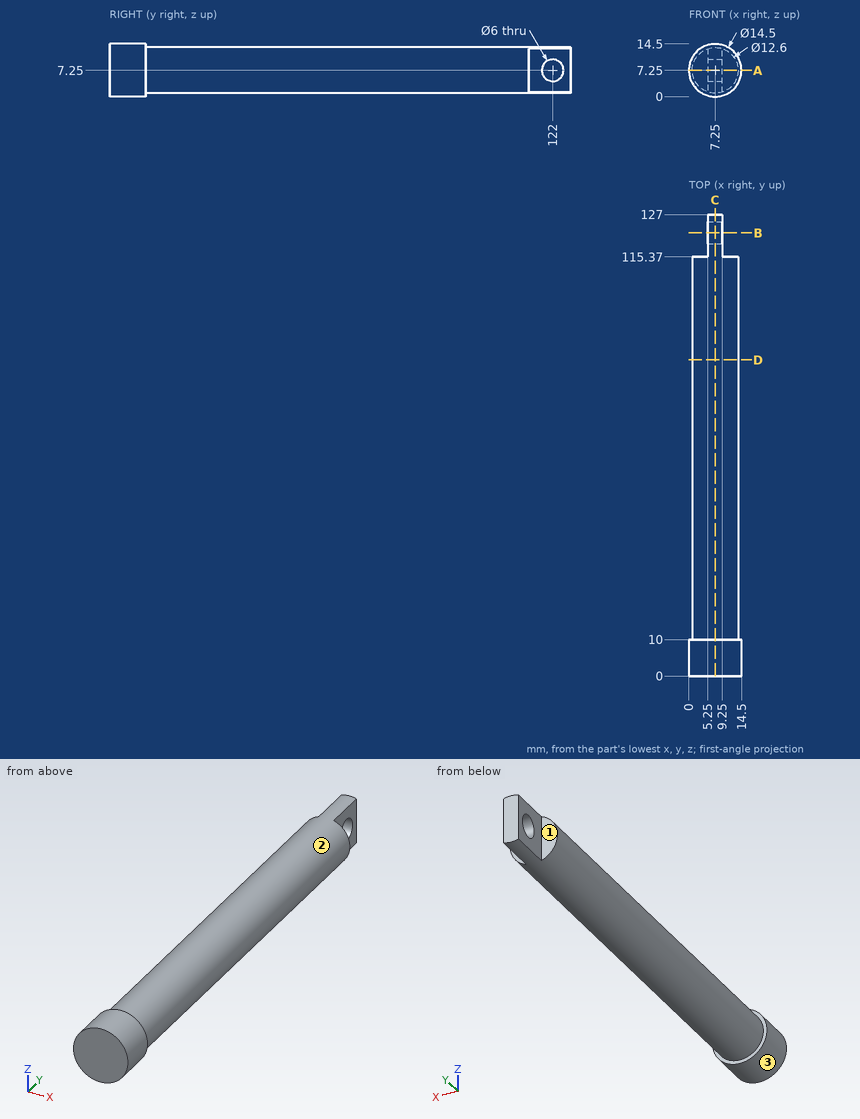
Geometry: see drawing. Coordinates: mm, zero at the bounding-box minimum. A direction names the side the tool comes from. Coordinates: 2 decimals unless noted, no trailing zeros. Loops run counter-clockwise (first coordinate to the right, second up) from the corner with the lowest first, then second, coordinate; pieces in that order, holes last. Notation, with made-up numbers: (46, 19.25) - (69, 19.25) arc R36 cw to (69, 55.25) - close; hole circle Ø2 at (0.25, -20.75). An arc over 180 degrees is marked (long way). Answer as CSV lines item,"result".
1. Section A-A (z = 7.25). Return loops of the section in (x, y).
Established:
outline,"(0, 0) - (14.5, 0) - (14.5, 10) - (13.55, 10) - (13.55, 115.37) - (9.25, 115.37) - (9.25, 119) - (5.25, 119) - (5.25, 115.37) - (0.95, 115.37) - (0.95, 10) - (0, 10) - close; (5.25, 125) - (9.25, 125) - (9.25, 127) - (5.25, 127) - close"
2. Contact query for flat-ended pins moving along their axis: pin 1 (5.5 mm diameter, centred on y = 122, z = 7.25, fed in from -X); pin 2 (6 mm diameter, centred on y = 118.5, z = 6, fed in from -X); pin 3 (2 mm diameter, centred on x = 12, z = 10, fed in from +Y); pin 4 (3 mm diameter, centred on x = 9, y = 86, fed in from +Z). Output: stop coordinate, or through.
Established:
pin 1,"passes through"
pin 2,"stops at x = 5.25"
pin 3,"stops at y = 115.37"
pin 4,"stops at z = 13.55"
3. Section B-B (y = 122). Return loops of the section in (x, z), then the cut area to 3 significant figures.
Established:
outline,"(5.25, 1.28) arc R6.3 ccw to (9.25, 1.28) - (9.25, 4.25) - (5.25, 4.25) - close; (5.25, 10.25) - (9.25, 10.25) - (9.25, 13.22) arc R6.3 ccw to (5.25, 13.22) - close"
area,"25.5 mm2"
4. Ray query, line 1 (Z direction, x = 7.3, y = 122); line 2 (Y direction, x = 10, z = 11.75); line 3 (Y direction, x = 2, z = 11.5). Return the intervals inside material, ascending.
Established:
line 1,"z = 0.95 to 4.25, 10.25 to 13.55"
line 2,"y = 0 to 115.37"
line 3,"y = 0 to 10"
5. Section D-D (y = 87). Return loops of the section in (x, z), then the cut area to 3 significant figures.
Established:
outline,"circle Ø12.6 at (7.25, 7.25)"
area,"125 mm2"
6. Section C-C (x = 7.25). Return loops of the section in (y, z), then the cut area to 3 significant figures.
Established:
outline,"(0, 0) - (10, 0) - (10, 0.95) - (127, 0.95) - (127, 13.55) - (10, 13.55) - (10, 14.5) - (0, 14.5) - close; hole circle Ø6 at (122, 7.25)"
area,"1,590 mm2"
7. Reachability of the marked faces 1, 2 and 3 from +Z, -Z, +X, -X, +Y, -Y: full face, straight path, thin tool, end or side. Return the list, or none.
Established:
face 1,"+Z, -Z, -X, +Y"
face 2,"+Y"
face 3,"+Y, -Y"
